The model under review builds one solid part; all positions refer to its coordinate system, in mm. Face numbers are marked on the shaded views. A direction names the side the tool comes from. Give positions to 0.01 mm unless a question says otherwise; leave off trailing zeros. Put each result on its own line as item: value. Start each with the question number.
```python
from build123d import *

# Parameters (mm, degrees)
FILLET1_R       = 0.2
FILLET2_R       = 0.25
HEX_2_DEPTH     = 2.5
THDSCHPAT_COUNT = 30
THDSCHPAT_PITCH = 0.779310345


with BuildPart() as part:
    # BodySke → Base-Revolve (revolve)
    with BuildSketch(Plane.XY):
        Polygon((0, 0), (0, 4.25), (5, 4.25), (5, 2.5), (29.555, 2.5), (30, 2.055), (30, 0), align=None)
    revolve(axis=Axis((-31.75, 0, 0), (1, 0, 0)))

    # Fillet1
    fillet1_edges = [part.edges().sort_by_distance(p)[0] for p in [
        (5, -2.5, 0),
    ]]
    fillet(fillet1_edges, radius=FILLET1_R)

    # Fillet2
    fillet2_edges = [part.edges().sort_by_distance(p)[0] for p in [
        (0, -4.25, 0),
    ]]
    fillet(fillet2_edges, radius=FILLET2_R)

    # Sketch2 → Hex-PreBroach (revolve, cut)
    with BuildSketch(Plane.XY):
        Polygon((0, 2.042), (2.5, 2.042), (3.67894925, 0), (0, 0), align=None)
    revolve(axis=Axis((0, 0, 0), (1, 0, 0)), mode=Mode.SUBTRACT)

    # Sketch3 → Hex 2 (cut)
    with BuildSketch(Plane(origin=(0, 0, 0), x_dir=(0, 0.5, 0.866025404), z_dir=(-1, 0, 0))):
        Polygon((1.17894925, 2.042), (-1.17894925, 2.042), (-2.357898499, 0), (-1.17894925, -2.042), (1.17894925, -2.042), (2.357898499, 0), align=None)
    extrude(amount=-HEX_2_DEPTH, mode=Mode.SUBTRACT)

    # ThdSchSke → ThreadSchematic (revolve, cut)
    with BuildSketch(Plane.XY):
        Polygon((7.4, -2.055), (7.088407645, -2.5), (7.088407645, -3.125), (7.711592355, -3.125), (7.711592355, -2.5), align=None)
    threadschematic = revolve(axis=Axis((-3.175, 0, 0), (1, 0, 0)), mode=Mode.SUBTRACT)

    # ThdSchPat: ThreadSchematic ×30
    with Locations(*[(i * THDSCHPAT_PITCH, 0, 0) for i in range(1, THDSCHPAT_COUNT)]):
        add(threadschematic, mode=Mode.SUBTRACT)


solid = part.part
```
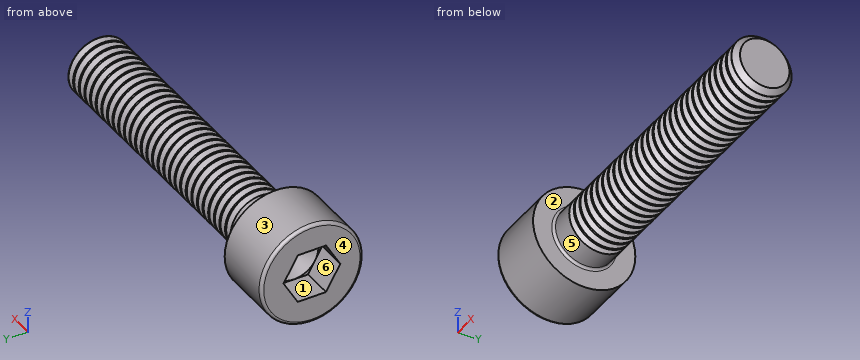
Item 1: To check wall thickness, follow L1, parallel to X at y = -2.25, z = -2; L2, parallel to Y at x = 1.5, z = -1.25; L3, parallel to Y at x = 1.75, z = 1.75. State the ranges of each line that lie inside material, in increasing order. Write a range as [from, to].
Item 2: Clearance check with flat-ended pins moving along their axes: pin 1 Ø1.5 at (x, z) = (7.5, 2.5) entering from +Y (3 decimals); pin 2 Ø2 at (x, y) = (22, 1) entering from -Z; pin 3 Ø5 at (x, y) = (22, 0.5) entering from +Z. State where each tip first meets the part, or that it passes through.
Item 3: Tool access review of the marked faces 4, 5 and 6: name each direction out of +Z, -Z, +X, -X, +Y, -Y from which nothing blocks a thin tool from reaching the whole face with its end or side.
Item 4: Draft analysis for pull direction Z (two halves, no side actions). For the marked faces 1, 2 and 3, state which applies: +Z half, -Z half, draft (parallel to the pull), parting line (faces both ways), or undercut.
Report:
1. L1: [0, 5]
1. L2: [-4.06, -1.64], [1.64, 4.06]
1. L3: [-3.87, -1.35], [1.35, 3.87]
2. pin 1: y = 1.755
2. pin 2: z = -2.5
2. pin 3: z = 2.5
3. face 4: +Z, -Z, -X, +Y, -Y
3. face 5: +X
3. face 6: -X
4. face 1: undercut
4. face 2: draft
4. face 3: parting line
